```python
from build123d import *

# Parameters (mm, degrees)
F0_R     = 19.20551
F0_R_2   = 9.580083
F1_DEPTH = 60
F2_R     = 24.322186
F2_W     = 39.359974
F2_H     = 24.98503
F3_DEPTH = 30
F4_R     = 5
F5_R     = 7.812244
F6_DEPTH = 45


with BuildPart() as f1:
    # F0 (on Front) → F1 (new body)
    with BuildSketch(Plane.XZ):
        with Locations((-77.851459, 19.139083)):
            Circle(F0_R)
        with Locations((-77.851459, 19.139083)):
            Circle(F0_R_2, mode=Mode.SUBTRACT)
    extrude(amount=F1_DEPTH)

    # F2 (on Top) → F3 (join)
    with BuildSketch(Plane.XY):
        with BuildLine():
            Line((10.089813, 0), (-60.415883, 0))
            Line((-60.415883, 0), (-60.415883, -59.699342))
            Line((-60.415883, -59.699342), (-35.088591, -59.699342))
            Line((-35.088591, -59.699342), (4.271383, -59.699342))
            Line((4.271383, -59.699342), (10.089813, -59.699342))
            ThreePointArc((10.089813, -59.699342), (39.939484, -29.849671), (10.089813, 0))
        make_face()
        with Locations((5.982686, -29.580405)):
            Circle(F2_R, mode=Mode.SUBTRACT)
        with Locations((-15.408604, -72.191857)):
            Rectangle(F2_W, F2_H)
    extrude(amount=F3_DEPTH)

    # F4
    f4_edges = [f1.edges().sort_by_distance(p)[0] for p in [
        (-15.408604, -84.684372, 30),
        (-15.408604, -84.684372, 0),
    ]]
    fillet(f4_edges, radius=F4_R)

    # F5 (on face) → F6 (cut)
    with BuildSketch(Plane.YZ.offset(4.271383)):
        with Locations((-72.369397, 15.990797)):
            Circle(F5_R)
    extrude(amount=-F6_DEPTH, mode=Mode.SUBTRACT)


solid = f1.part
```
Geometry check sheet. Reference: the model listing, model coordinates, mm. A direction names the side the tool comes from. Give positions to 0.01 mm unless a question says otherwise; leave off trailing zeros. Loops run counter-clockwise (first coordinate to the right, second up) from the corner with the lowest first, then second, coordinate; pieces in that order, holes last. Notation, with made-up numbers: (-26.75, 65.25) - (-14.75, 65.25) arc R17 cw to (-14.75, 70.25) - close; hole circle Ø8 at (69, 66.5). An arc over 180 degrees is marked (long way). Use CSV: the item, a comma, the result in double quotes. Start each with the question number.
Q1. Release check for a two-part mould opening along X. For faces 4 (the face through (-60.416, -29, 5)), 5 (the face through (4.271, -72, 8)), 6 (the face through (7, -59.699, 15)) record: +X half, -X half, draft (parallel to the pull), parting line (faces both ways), or undercut.
Q2. Section check D-D, the plane y = -72. Record the cut outline in (x, z).
Q3. Section check A-A, the plane z = 14. Record the cut outline in (x, y), and give its area (3 significant figures).
Q4. Access from +Z, -Z, +X, -X, +Y, -Y to the whole of each face (thin tool, end or side, straight path). Record for faces 1 (the face through (-22, -39, 30)), 2 (the face through (-87, -60, 15)), 3 (the face through (2.816, -5.465, 14.79)).
Q5. Section check B-B, the plane x = -83. Record the cut outline in (y, z).
Q6. Section check C-C, the plane y = -26.5. Record the cut outline in (x, z).
Q7. Go/stop test with flat-tipped pins: pin 1 Ø10 at (x, z) = (-76.5, 18.5) entering from -Y; pin 2 Ø12.5 at (y, z) = (-75, 21) entering from +X; pin 3 Ø6 at (y, z) = (-55, 28.5) entering from -X; pin 4 Ø3 at (x, z) = (6.5, 22.5) entering from -Y. Record where each tip stops, or that it passes through.
Q8. Scan lines: probe 1 along X at (y, z) = (-45, 29.5); probe 2 along X at (y, z) = (-46.5, 21.5); probe 3 along Y at (x, z) = (-16.5, 12). Record each from-to range of solid material in increasing order. Write a range as from..to.
Findings below:
1,face 4,"undercut"
1,face 5,"+X half"
1,face 6,"draft"
2,outline,"(-35.09, 0) - (4.27, 0) - (4.27, 8.19) - (-35.09, 8.19) - close; (-35.09, 23.79) - (4.27, 23.79) - (4.27, 30) - (-35.09, 30) - close"
3,outline,"(-96.36, -60) - (-85.94, -60) - (-85.94, 0) - (-96.36, 0) - close; (-69.77, -60) - (-59.35, -60) - (-59.35, -59.7) - (-35.09, -59.7) - (-35.09, -64.82) - (4.27, -64.82) - (4.27, -59.7) - (10.09, -59.7) arc R29.85 ccw to (10.09, 0) - (-69.77, 0) - close; (-35.09, -84.68) - (4.27, -84.68) - (4.27, -79.92) - (-35.09, -79.92) - close; hole circle Ø48.64 at (5.98, -29.58)"
3,area,"5,330 mm^2"
4,face 1,"+Z, +X, +Y, -Y"
4,face 2,"+Z, -Z, -X, -Y"
4,face 3,"+Z, -Z"
5,outline,"(-60, 0.64) - (0, 0.64) - (0, 11.06) - (-60, 11.06) - close; (-60, 27.22) - (0, 27.22) - (0, 37.64) - (-60, 37.64) - close"
6,outline,"(-60.42, 0) - (-18.14, 0) - (-18.14, 30) - (-60.42, 30) - (-60.42, 27.19) arc R19.21 ccw (long way) to (-60.42, 11.09) - close; (30.11, 0) - (39.75, 0) - (39.75, 30) - (30.11, 30) - close; hole circle Ø19.16 at (-77.85, 19.14)"
7,pin 1,"passes through"
7,pin 2,"stops at x = 4.27"
7,pin 3,"stops at x = -95.97"
7,pin 4,"stops at y = -59.7"
8,probe 1,"x = -94.02..-61.68, -60.42..-12.83, 24.79..35.81"
8,probe 2,"x = -96.91..-87.14, -68.57..-11.49, 23.46..34.86"
8,probe 3,"y = -84.68..-79.09, -65.65..-38.86, -20.3..0"
